Autodesk Inventor part; units mm, degrees
ref_plane "YZ Plane" through (0, 0, 0) normal (1, 0, 0) x (0, 1, 0)
ref_plane "XZ Plane" through (0, 0, 0) normal (0, 1, 0) x (-1, 0, 0)
ref_plane "XY Plane" through (0, 0, 0) normal (0, 0, 1) x (1, 0, 0)
sketch "Sketch1" plane through (0, 0, 0) normal (0, 0, 1) x (1, 0, 0)
  circle A0 centre (0, 0) radius 40
  circle A1 centre (0, 0) radius 5.375
  dimension "d0" = 80
  dimension "d1" = 10.75
extrude "Extrusion1" add sketch "Sketch1" along normal blind 4
sketch "Sketch5" plane through (0, 0, 4) normal (0, 0, 1) x (1, 0, 0)
  point P0 (0, 0)
sketch "Sketch7" plane through (0, 0, 4) normal (0, 0, 1) x (1, 0, 0)
  line L0 (-9.9, 10) -> (9.9, 10)
  line L1 (9.9, 10) -> (9.9, -30.6)
  line L2 (9.9, -30.6) -> (-9.9, -30.6)
  line L3 (-9.9, -30.6) -> (-9.9, 10)
  circle A0 centre (0, 0) radius 5.375
  dimension "d19" = 19.8
  dimension "d20" = 40.6
  dimension "d21" = 10
  dimension "d22" = 9.9
extrude "Extrusion5" cut sketch "Sketch7" against normal blind 4
properties part number "base22"
The listing builds one solid part. Answer for the finished solid, in the listing's coordinates (mm). A direction names the side the tool comes from. Give positions to 0.01 mm unless a question says otherwise; leave off trailing zeros. Loops run counter-clockwise (first coordinate to the right, second up) from the corner with the lowest first, then second, coordinate; pieces in that order, holes last. Notation, with made-up numbers: (-34, -23.75) - (24, -23.75) arc R11 cw to (24, -19.75) - close; hole circle Ø1 at (72, 64.5). An arc over 180 degrees is marked (long way). Write each question's results on one line, items separated by ' | '.
1. Find section B-B, the plane x = 0. Write down the section's boundary in (y, z).
Resolved:
outline: (-40, 0) - (-30.6, 0) - (-30.6, 4) - (-40, 4) - close; (10, 0) - (40, 0) - (40, 4) - (10, 4) - close
2. Find section A-A, the plane y = 0. Write down the section's boundary in (x, z), then the cut area to 3 significant figures.
Resolved:
outline: (-40, 0) - (-9.9, 0) - (-9.9, 4) - (-40, 4) - close; (9.9, 0) - (40, 0) - (40, 4) - (9.9, 4) - close | area: 241 mm^2
3. For a pull along Y with two mould halves and no side action, classify faces 3 (the face through (17, 1, 4)), 4 (the face through (0, -30.6, 2)), 5 (the face through (-8.67, 39.05, 1.97)) as +Y half, -Y half, draft (parallel to the pull), parting line (faces both ways), or undercut.
Resolved:
face 3: draft | face 4: undercut | face 5: parting line
4. Flat-ended cylindrical pins translate along their axes: P1, Ø1, axis at y = -4.5, z = 2.5, coming from the +X side; P2, Ø1.2, axis at y = -14.5, z = 2.5, coming from the +X side; P3, Ø1.2, axis at x = 2, z = 1, coming from the +Y side. Find the tip coordinate at first contact, or state that the pin passes through.
Resolved:
P1: stops at x = 39.8 | P2: stops at x = 37.51 | P3: stops at y = 39.98
5. Find section C-C, the plane z = 2.65. Write down the section's boundary in (x, y).
Resolved:
outline: circle Ø80 at (0, 0); hole (-9.9, -30.6) - (9.9, -30.6) - (9.9, 10) - (-9.9, 10) - close
6. Find section D-D, the plane y = 22. Write down the section's boundary in (x, z), then the cut area to 3 significant figures.
Resolved:
outline: (-33.41, 0) - (33.41, 0) - (33.41, 4) - (-33.41, 4) - close | area: 267 mm^2
7. Consider probe 1 along X at (y, z) = (-1, 2); probe 2 along X at (y, z) = (-2, 1.8); probe 3 along Y at (x, z) = (-3, 0.45). Determine where each line is inside the solid, lowest interval first. Write a range as from..to.
Resolved:
probe 1: x = -39.99..-9.9, 9.9..39.99 | probe 2: x = -39.95..-9.9, 9.9..39.95 | probe 3: y = -39.89..-30.6, 10..39.89
8. Which of the six approach directions +Z, -Z, +X, -X, +Y, -Y give full straight-line access (tool end or side, diameter ignored) to faces 1 (the face through (0, 10, 2)), 2 (the face through (17, 1, 0))?
Resolved:
face 1: +Z, -Z | face 2: -Z, +X, -X, +Y, -Y
